The model under review builds one solid part; all positions refer to its coordinate system, in mm. Face numbers are marked on the shaded views. A direction names the side the tool comes from. Round coordinates to 2 decimals unless told otherwise and drop trailing zeros. Loops run counter-clockwise (first coordinate to the right, second up) from the corner with the lowest first, then second, coordinate; pieces in that order, holes last. Notation, with made-up numbers: (43.25, -3) -> (72.25, -3) arc R28 cw to (72.25, 16) -> close; hole circle Ø2 at (-1, -4.75). An arc over 180 degrees is marked (long way). Write each question's results on one line, items separated by ' | '. Start each with the question number.
Item 1: We need section B-B (x = 26). Give the boundary of the cut face in (y, z).
Item 2: Clearance check with a flat-ended pin moving along its axis: pin 1 Ø6 at (x, z) = (136.5, -60) entering from -Y. State where the tip first meets the part, or that it passes through.
Item 3: Tool access review of the marked faces 1 and 2: name each direction out of +Z, -Z, +X, -X, +Y, -Y from which nothing blocks a thin tool from reaching the whole face with its end or side.
Item 4: We need section A-A (y = 95). Give the boundary of the cut face in (x, z), and give its area (4 significant figures).
Item 5: We need section C-C (z = -40). Give the boundary of the cut face in (x, y).
Item 6: Mouldability with a two-part tool opening along Z and no side actions: class the marked faces 3, 4 and 5 as pulls with the +Z half, pulls with the -Z half, needs draft (parallel to the pull), parting line crosses it, or undercut.
Item 7: For L1, parallel to Z at x = -4, y = 87.5; L2, parallel to X at y = -111.5, z = 92; L3, parallel to Y at x = -17, z = -85.5, list the stretches that pass through material, from the lowest coordinate up. Write a range as from..to.
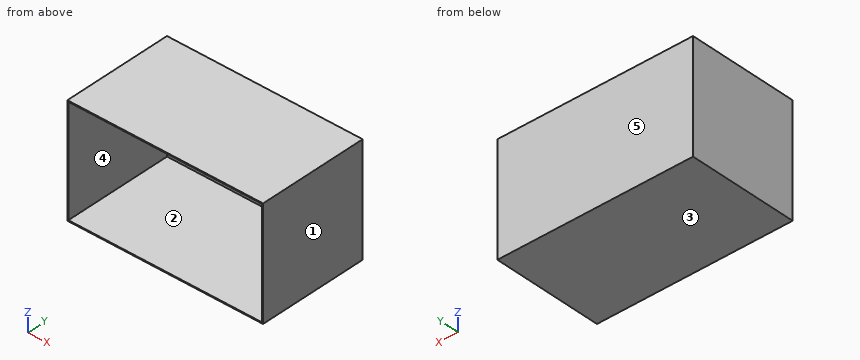
from build123d import *

# Parameters (mm, degrees)
F0_W      = 480
F0_H      = 270
F1_DEPTH  = 135
F1_FACE_W = 480
F1_FACE_H = 270
F2_DEPTH  = 135
F3_T      = -2.5


with BuildPart() as f1:
    # F0 (on Top) → F1 (new body)
    with BuildSketch(Plane.XY):
        Rectangle(F0_W, F0_H)
    extrude(amount=F1_DEPTH)

    # F1_face (on face) → F2 (join)
    with BuildSketch(Plane(origin=(0, 0, 0), x_dir=(1, 0, 0), z_dir=(0, 0, -1))):
        Rectangle(F1_FACE_W, F1_FACE_H)
    extrude(amount=F2_DEPTH)

    # F3
    f3_openings = [f1.faces().sort_by_distance(p)[0] for p in [
        (0, -135, 0),
    ]]
    offset(amount=F3_T, openings=f3_openings)


solid = f1.part
Here are the results:
1) outline: (-135, -135) -> (135, -135) -> (135, 135) -> (-135, 135) -> (-135, 132.5) -> (132.5, 132.5) -> (132.5, -132.5) -> (-135, -132.5) -> close
2) pin 1: stops at y = 132.5
3) face 1: +Z, -Z, +X, +Y, -Y | face 2: -Y
4) outline: (-240, -135) -> (240, -135) -> (240, 135) -> (-240, 135) -> close; hole (-237.5, -132.5) -> (237.5, -132.5) -> (237.5, 132.5) -> (-237.5, 132.5) -> close | area: 3,725 mm2
5) outline: (-240, -135) -> (-237.5, -135) -> (-237.5, 132.5) -> (237.5, 132.5) -> (237.5, -135) -> (240, -135) -> (240, 135) -> (-240, 135) -> close
6) face 3: pulls with the -Z half | face 4: undercut | face 5: needs draft
7) L1: z = -135..-132.5, 132.5..135 | L2: x = -240..-237.5, 237.5..240 | L3: y = 132.5..135
